```python
from build123d import *

# Parameters (mm, degrees)
SKETCH1_R           = 12.5
BOSS_EXTRUDE1_DEPTH = 10
FILLET1_R           = 2.5
SKETCH2_R           = 8
BOSS_EXTRUDE2_DEPTH = 100
SKETCH3_R           = 3
CUT_EXTRUDE1_DEPTH  = 50


with BuildPart() as part:
    # Sketch1 → Boss-Extrude1 (new body)
    with BuildSketch(Plane(origin=(0, 0, 0), x_dir=(1, 0, 0), z_dir=(0, 1, 0))):
        with Locations(Location((0, 0, 0), (0, 0, 270))):
            Circle(SKETCH1_R)
    extrude(amount=BOSS_EXTRUDE1_DEPTH)

    # Fillet1
    fillet1_edges = [part.edges().sort_by_distance(p)[0] for p in [
        (0, 0, -12.5),
    ]]
    fillet(fillet1_edges, radius=FILLET1_R)

    # Sketch2 → Boss-Extrude2 (add)
    with BuildSketch(Plane(origin=(0, 10, 0), x_dir=(1, 0, 0), z_dir=(0, 1, 0))):
        with Locations(Location((0, 0, 0), (0, 0, 270))):
            Circle(SKETCH2_R)
    extrude(amount=BOSS_EXTRUDE2_DEPTH)

    # Sketch3 → Cut-Extrude1 (cut, symmetric)
    with BuildSketch(Plane.XY):
        with Locations(Location((0, 104, 0), (0, 0, 90.000000025))):
            Circle(SKETCH3_R)
    extrude(amount=CUT_EXTRUDE1_DEPTH, both=True, mode=Mode.SUBTRACT)


solid = part.part
```
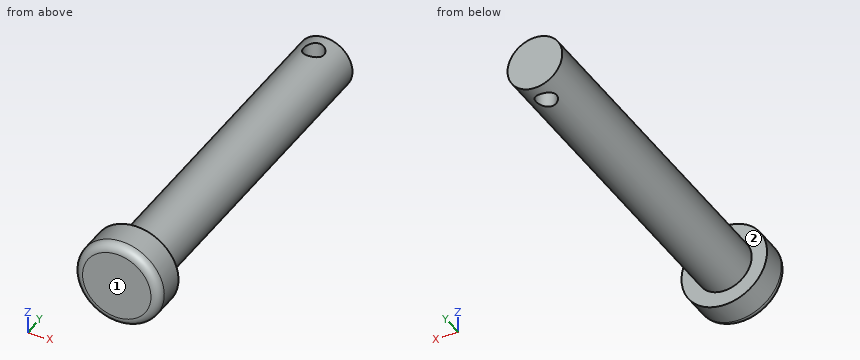
Part model, mm, in its own coordinate system. Face numbers are marked on the shaded views. A direction names the side the tool comes from. Coordinates: 2 decimals unless noted, no trailing zeros. Order: outer loops, then holes, each group sorted by start corner. A loop starts at its lowest first (then second) coordinate and runs counter-clockwise, first axis right, second up. Notation, with made-up numbers: (13.5, 72.5) -> (32.5, 72.5) arc R13 ccw to (32.5, 84.5) -> close; hole circle Ø10 at (41, 27). An arc over 180 degrees is marked (long way). Put each result on its own line as item: value. Start each with the question number.
(1) Band-saw the part on C-C (y = 104). Give the cut face in (x, z), then the cut area to 3 significant figures.
(2) Probe line 1 along Y through (x, z) = (0, 2.5); line 2 along Z through (x, y) = (-0.25, 73); line 3 along X through (y, z) = (104, 2.25). List the from-to ranges inside material, lowest first. Write a range as [from, to].
(3) Band-saw the part on B-B (y = 14). Give the cut face in (x, z), then the cut area to 3 significant figures.
(4) Which spindle directions (+Z, -Z, +X, -X, +Y, -Y) get a long thin tool onto all of the face, cutting with end or side? Do the marked faces 1 and 2. Say none if no direction does.
(5) Band-saw the part on A-A (z = 0). Give the cut face in (x, y), then the cut area to 3 significant figures.
(6) Pin check, flat tips, straight feed: pin 1 Ø10 at (y, z) = (83.5, 9.5) entering from +X; pin 2 Ø12 at (x, y) = (-2, 81.5) entering from -Z; pin 3 Ø8 at (x, y) = (-2.5, 41.5) entering from +Z. Stop position of each tip, or through.
Determined:
1. outline: (-3, -7.42) -> (-3, 7.42) arc R8 ccw to start; (3, -7.42) arc R8 ccw to (3, 7.42) -> close
1. area: 107 mm²
2. line 1: y = [0, 101], [107, 110]
2. line 2: z = [-8, 8]
2. line 3: x = [-7.68, -3], [3, 7.68]
3. outline: circle Ø16 at (0, 0)
3. area: 201 mm²
4. face 1: +Z, -Z, +X, -X, -Y
4. face 2: +Y
5. outline: (-12.5, 2.5) arc R2.5 ccw to (-10, 0) -> (10, 0) arc R2.5 ccw to (12.5, 2.5) -> (12.5, 10) -> (8, 10) -> (8, 110) -> (-8, 110) -> (-8, 10) -> (-12.5, 10) -> close; hole circle Ø6 at (0, 104)
5. area: 1,820 mm²
6. pin 1: stops at x = 6.61
6. pin 2: stops at z = -8
6. pin 3: stops at z = 8
